Autodesk Inventor part; units mm, degrees
ref_plane "YZ Plane" through (0, 0, 0) normal (1, 0, 0) x (0, 1, 0)
ref_plane "XZ Plane" through (0, 0, 0) normal (0, 1, 0) x (-1, 0, 0)
ref_plane "XY Plane" through (0, 0, 0) normal (0, 0, 1) x (1, 0, 0)
sketch "Sketch1" plane through (0, 0, 0) normal (0, 1, 0) x (-1, 0, 0)
  line L0 (-23, 13) -> (23, 13)
  line L1 (23, 13) -> (23, -13)
  line L2 (23, -13) -> (-23, -13)
  line L3 (-23, -13) -> (-23, 13)
  line L4 (-23, 13) -> (23, -13) construction
  line L5 (23, 13) -> (-23, -13) construction
  line L6 (0, 0) -> (-11, 0)
  circle A0 centre (-11, 0) radius 8.75
  line L7 (0, 0) -> (11, 0)
  circle A1 centre (11, 0) radius 8.75
  dimension "d0" = 46
  dimension "d1" = 26
  dimension "d2" = 11
  dimension "d3" = 17.5
  dimension "d4" = 11
  dimension "d5" = 17.5
extrude "Extrusion1" add sketch "Sketch1" along normal blind 5
sketch "Sketch3" plane through (-23, 0, 13) normal (0, 0, 1) x (1, 0, 0)
  line L0 (46, 0) -> (0, 0)
  line L1 (46, 0) -> (46, 5)
  line L2 (0, 5) -> (46, 5)
  line L3 (0, 0) -> (0, 5)
  point P0 (23, 0)
extrude "Extrusion2" add sketch "Sketch3" along normal blind 5
sketch "Sketch2" plane through (0, 5, 0) normal (0, 1, 0) x (1, 0, 0)
  circle A0 centre (-11, 0) radius 8.75
  circle A1 centre (11, 0) radius 8.75
  line L0 (23, 13) -> (23, -18)
  line L1 (23, 13) -> (-23, 13)
  line L2 (-23, 13) -> (-23, -18)
  line L3 (23, 13) -> (-23, 13)
  line L4 (0, 13) -> (0, 10)
  line L5 (-4, 9) -> (4, 9)
  line L6 (4, 9) -> (4, 11)
  line L7 (4, 11) -> (-4, 11)
  line L8 (-4, 11) -> (-4, 9)
  line L9 (-4, 9) -> (4, 11) construction
  line L10 (4, 9) -> (-4, 11) construction
  line L11 (23, -18) -> (-23, -18)
  line L12 (23, -18) -> (-23, -18)
  line L13 (0, -18) -> (0, -15)
  line L14 (-4, -16) -> (4, -16)
  line L15 (4, -16) -> (4, -14)
  line L16 (4, -14) -> (-4, -14)
  line L17 (-4, -14) -> (-4, -16)
  line L18 (-4, -16) -> (4, -14) construction
  line L19 (4, -16) -> (-4, -14) construction
  line L20 (-23, 13) -> (-23, -18)
  line L21 (-23, -18) -> (-23, -13)
  line L22 (-23, -13) -> (-20, -13)
  line L23 (-21, -16) -> (-19, -16)
  line L24 (-19, -16) -> (-19, -10)
  line L25 (-19, -10) -> (-21, -10)
  line L26 (-21, -10) -> (-21, -16)
  line L27 (-21, -16) -> (-19, -10) construction
  line L28 (-19, -16) -> (-21, -10) construction
  point P0 (0, 0)
  dimension "d8" = 3
  dimension "d9" = 8
  dimension "d10" = 2
  dimension "d16" = 3
  dimension "d17" = 8
  dimension "d18" = 2
  dimension "d19" = 5
  dimension "d20" = 3
  dimension "d21" = 2
  dimension "d22" = 6
extrude "Extrusion3" cut sketch "Sketch2" against normal blind 5 contours L7 L6 L5 L8 | L26 L25 L24 L23 | L14 L17 L16 L15
sketch "Sketch4" plane through (0, 5, 0) normal (0, 1, 0) x (1, 0, 0)
  line L0 (4, 11) -> (4, 9)
  line L1 (4, 9) -> (-4, 9)
  line L2 (-4, 9) -> (-4, 11)
  line L3 (-4, 11) -> (4, 11)
  line L4 (-19, -10) -> (-19, -16)
  line L5 (-19, -16) -> (-21, -16)
  line L6 (-21, -16) -> (-21, -10)
  line L7 (-21, -10) -> (-19, -10)
  line L8 (4, -14) -> (4, -16)
  line L9 (4, -16) -> (-4, -16)
  line L10 (-4, -16) -> (-4, -14)
  line L11 (-4, -14) -> (4, -14)
  circle A0 centre (-11, 0) radius 8.75
  circle A1 centre (11, 0) radius 8.75
  line L12 (23, 13) -> (23, -18)
  line L13 (23, 13) -> (-23, 13)
  line L14 (-23, 13) -> (-23, -18)
  line L15 (23, -18) -> (-23, -18)
  point P0 (0, 0)
extrude "Extrusion4" add sketch "Sketch4" along normal blind 3
sketch "Sketch5" plane through (0, 8, 0) normal (0, 1, 0) x (1, 0, 0)
  circle A0 centre (11, 0) radius 8.75
  circle A1 centre (-11, 0) radius 8.75
  line L0 (4, -16) -> (-4, -16)
  line L1 (-4, -16) -> (-4, -14)
  line L2 (-4, -14) -> (4, -14)
  line L3 (4, -14) -> (4, -16)
  line L4 (4, 9) -> (-4, 9)
  line L5 (-4, 9) -> (-4, 11)
  line L6 (-4, 11) -> (4, 11)
  line L7 (4, 11) -> (4, 9)
  line L8 (-19, -16) -> (-21, -16)
  line L9 (-21, -16) -> (-21, -10)
  line L10 (-21, -10) -> (-19, -10)
  line L11 (-19, -10) -> (-19, -16)
  line L12 (23, -18) -> (23, 13)
  line L13 (23, 13) -> (-23, 13)
  line L14 (-23, 13) -> (-23, -18)
  line L15 (-23, -18) -> (23, -18)
  line L16 (-20.5, -9.5) -> (-1.5, -9.5)
  line L17 (-1.5, -9.5) -> (-1.5, 9.5)
  line L18 (-1.5, 9.5) -> (-20.5, 9.5)
  line L19 (-20.5, 9.5) -> (-20.5, -9.5)
  line L20 (-20.5, -9.5) -> (-1.5, 9.5) construction
  line L21 (-1.5, -9.5) -> (-20.5, 9.5) construction
  line L22 (1.5, -9.5) -> (20.5, -9.5)
  line L23 (20.5, -9.5) -> (20.5, 9.5)
  line L24 (20.5, 9.5) -> (1.5, 9.5)
  line L25 (1.5, 9.5) -> (1.5, -9.5)
  line L26 (1.5, -9.5) -> (20.5, 9.5) construction
  line L27 (20.5, -9.5) -> (1.5, 9.5) construction
  point P0 (0, 0)
  dimension "d27" = 19
  dimension "d28" = 19
  dimension "d29" = 19
  dimension "d30" = 19
extrude "Extrusion5" cut sketch "Sketch5" against normal blind 5 contours A0 | A1 | L7 L24 L23 L22 L25 L4 | L4 L25 L24 L7 | L17 L16 L19 L18 L5 L4 | L4 L5 L18 L17
properties part number "buttons"
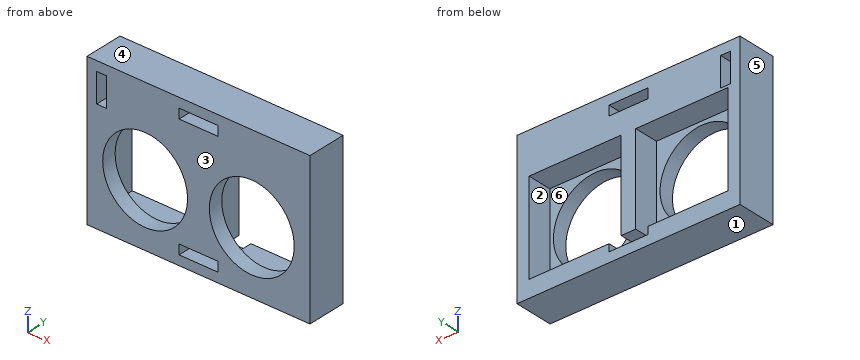
The model under review builds one solid part; all positions refer to its coordinate system, in mm. Face numbers are marked on the shaded views. A direction names the side the tool comes from. Give positions to 0.01 mm unless a question says otherwise; leave off trailing zeros. Write each loop counter-clockwise with the first axis right and the second up, starting at its lowest first coordinate (ties: lowest second). Pieces come first, ordered by that corner, then holes. Notation, with made-up numbers: M 46,-8.75 L 100,-8.75 A8 ccw 100,-4.75 Z; hole C -34.5,78 d5. An arc over 180 degrees is marked long. Write item = value, one per line. Start each with the question number.
Q1. We need section C-C (x = 11). State the section outline as (y, z) points, plus the area to 4 significant figures.
Q2. We need section D-D (y = 4.75). State the section outline as (x, z) points.
Q3. Mouldability with a two-part tool opening along Z and no side actions: class the marked faces 1, 2, 3 and 4 as released by +Z, released by -Z, zero draft, split by the parting line, or undercut.
Q4. We need section A-A (y = 2). State the section outline as (x, z) points.
Q5. Machinability: for the marked faces 5 and 6, which of the approach directions +Z, -Z, +X, -X, +Y, -Y give a long, thin tool a straight path to every point of the face, cutting with its end or side? Answer none if there is none.
Q6. We need section B-B (z = 0). State the section outline as (x, y) points.
Q7. For line 1 (Z direction, x = 2.5, y = 4.5); line 2 (X direction, y = 1.3, z = 0); line 3 (Z direction, x = -11, y = 3.5), list the stretches that pass through material, from the lowest coordinate up.
Q8. Clearance check with flat-ended pins moving along their axes: pin 1 (8 mm diameter, centred on x = 14.5, z = -9, fed in from +Y); pin 2 (1.5 mm diameter, centred on x = -17.5, z = -6.5, fed in from +Y). State where each tip first meets the part, or that it passes through.
Result set:
q1.outline = M 0,-13 L 8,-13 L 8,-9.5 L 3,-9.5 L 3,-8.75 L 0,-8.75 Z; M 0,8.75 L 3,8.75 L 3,9.5 L 8,9.5 L 8,18 L 0,18 Z
q1.area = 100.5 mm2
q2.outline = M -23,-13 L 23,-13 L 23,18 L -23,18 Z; hole M -21,10 L -19,10 L -19,16 L -21,16 Z; hole M -20.5,-9.5 L -4,-9.5 L -4,-11 L 4,-11 L 4,-9.5 L 20.5,-9.5 L 20.5,9.5 L 1.5,9.5 L 1.5,-9 L -1.5,-9 L -1.5,9.5 L -20.5,9.5 Z; hole M -4,14 L 4,14 L 4,16 L -4,16 Z
q3.face_1 = released by -Z
q3.face_2 = undercut
q3.face_3 = zero draft
q3.face_4 = released by +Z
q4.outline = M -23,-13 L 23,-13 L 23,18 L -23,18 Z; hole M -21,10 L -19,10 L -19,16 L -21,16 Z; hole C -11,0 d17.5; hole M -4,-11 L 4,-11 L 4,-9 L -4,-9 Z; hole M -4,14 L 4,14 L 4,16 L -4,16 Z; hole C 11,0 d17.5
q5.face_5 = +Z, -Z, -X, +Y, -Y
q5.face_6 = +Y
q6.outline = M -23,0 L -19.75,0 L -19.75,3 L -20.5,3 L -20.5,8 L -23,8 Z; M -2.25,0 L 2.25,0 L 2.25,3 L 1.5,3 L 1.5,8 L -1.5,8 L -1.5,3 L -2.25,3 Z; M 19.75,0 L 23,0 L 23,8 L 20.5,8 L 20.5,3 L 19.75,3 Z
q7.line_1 = -13 to -11, 9.5 to 14, 16 to 18
q7.line_2 = -23 to -19.75, -2.25 to 2.25, 19.75 to 23
q7.line_3 = -13 to -9.5, 9.5 to 18
q8.pin_1 = 8
q8.pin_2 = 3
